Can you work these out from the model? Positions are in its coordinate system, mm. Face numbers are marked on the shaded views. A direction names the side the tool comes from. Give positions to 0.01 mm unless a question says otherwise; leave off trailing zeros. Order: outer loops, then holes, each group sorted by start corner. A loop starts at its lowest first (then second) coordinate and runs counter-clockwise, first axis right, second up. Notation, with made-up numbers: (55, -8.5) - (114, -8.5) arc R33 cw to (114, 21.5) - close; hole circle Ø6 at (-34.5, -6). An arc over 180 degrees is marked (long way). Answer as CSV lines item,"result".
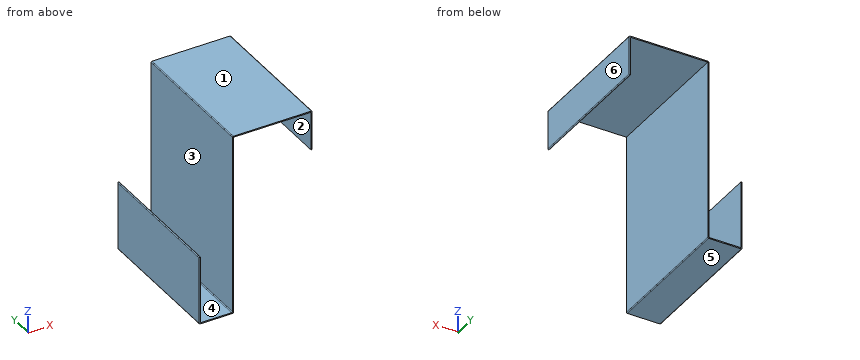
```python
from build123d import *

# Parameters (mm, degrees)
F1_DEPTH = 80
F2_R     = 1


with BuildPart() as f1:
    # F0 (on Front) → F1 (new body, symmetric)
    with BuildSketch(Plane.XZ):
        Polygon((-155.952706, -85), (-157.252706, -85), (-157.252706, -165), (-117.252706, -165), (-117.252706, 45), (-27.252706, 45), (-27.252706, 0), (-25.952706, 0), (-25.952706, 46.3), (-118.552706, 46.3), (-118.552706, -163.7), (-155.952706, -163.7), align=None)
    extrude(amount=F1_DEPTH, both=True)

    # F2
    f2_edges = [f1.edges().sort_by_distance(p)[0] for p in [
        (-118.552706, 0, 46.3),
        (-25.952706, 0, 46.3),
        (-117.252706, 0, -165),
        (-157.252706, 0, -165),
        (-25.952706, 0, 0),
        (-157.252706, 0, -85),
        (-155.952706, 0, -163.7),
        (-118.552706, 0, -163.7),
    ]]
    fillet(f2_edges, radius=F2_R)


solid = f1.part
```
1) Which directions (+Z, -Z, +X, -X, +Y, -Y) give clear straight access to the entire face, cutting with the end or side of a thin tool? Please do the marked faces 1, 2 and 3.
Answer block:
face 1,"+Z, +X, -X, +Y, -Y"
face 2,"-Z, +Y, -Y"
face 3,"+Z, +Y, -Y"
2) I want a section at D-D on z = -27. Write out the boundary of the cut face in (x, y).
Answer block:
outline,"(-118.55, -80) - (-117.25, -80) - (-117.25, 80) - (-118.55, 80) - close"
3) I want a section at C-C on x = -83. Write out the boundary of the cut face in (y, z), plus the area to 3 significant figures.
Answer block:
outline,"(-80, 45) - (80, 45) - (80, 46.3) - (-80, 46.3) - close"
area,"208 mm2"
4) If we mould it in two halves opening along X, with no side actions, what happens to the marked faces 4, 5 and 6? For each: +X half, -X half, draft (parallel to the pull), parting line (faces both ways), or undercut.
Answer block:
face 4,"undercut"
face 5,"draft"
face 6,"+X half"
5) I need wall thicknesses on line 1 along X through (y, z) = (9, 2); line 2 along X through (y, z) = (-35, -133.5); line 3 along X through (y, z) = (-63.5, -35). Which ranges of each line are inside material? Lowest first, please. Write a range as [from, to].
Answer block:
line 1,"[-118.55, -117.25], [-27.25, -25.95]"
line 2,"[-157.25, -155.95], [-118.55, -117.25]"
line 3,"[-118.55, -117.25]"
6) I want a section at B-B on y = 44.5. Write out the boundary of the cut face in (x, z), plus the area to 3 significant figures.
Answer block:
outline,"(-157.25, -164) arc R1 ccw to (-156.25, -165) - (-118.25, -165) arc R1 ccw to (-117.25, -164) - (-117.25, 45) - (-27.25, 45) - (-27.25, 0) - (-26.95, 0) arc R1 ccw to (-25.95, 1) - (-25.95, 45.3) arc R1 ccw to (-26.95, 46.3) - (-117.55, 46.3) arc R1 ccw to (-118.55, 45.3) - (-118.55, -162.7) arc R1 cw to (-119.55, -163.7) - (-154.95, -163.7) arc R1 cw to (-155.95, -162.7) - (-155.95, -85) - (-156.25, -85) arc R1 ccw to (-157.25, -86) - close"
area,"604 mm2"
7) I want a section at A-A on z = -150.5. Write out the boundary of the cut face in (x, y), plus the area to 3 significant figures.
Answer block:
outline,"(-157.25, -80) - (-155.95, -80) - (-155.95, 80) - (-157.25, 80) - close; (-118.55, -80) - (-117.25, -80) - (-117.25, 80) - (-118.55, 80) - close"
area,"416 mm2"
8) I'm going to push flat-ended pins straight in: P1, Ø3, axis at x = -124.5, y = 46, coming from the +Z side; P2, Ø13.5, axis at y = -8.5, z = 26, coming from the -X side; P3, Ø1.5, axis at y = 40.5, z = -33.5, coming from the +X side. Where does each tip first touch, or does it pass through?
Answer block:
P1,"z = -163.7"
P2,"x = -118.55"
P3,"x = -117.25"
